For this review, take the finished solid that the model builds, in its own axes (mm). A direction names the side the tool comes from. Round coordinates to 2 decimals unless told otherwise and drop trailing zeros. Order: outer loops, then holes, each group sorted by start corner. A loop starts at its lowest first (then second) coordinate and runs counter-clockwise, first axis right, second up. Notation, with made-up numbers: M -25.75,78.25 L 16.25,78.25 A34 ccw 16.25,111.25 Z; hole C -26,-5 d9. An arc over 180 degrees is marked long. Write item = value, one per line. Start each with the question number.
from build123d import *

# Parameters (mm, degrees)
F0_R     = 1.75
F1_DEPTH = 2


with BuildPart() as f1:
    # F0 (on Front) → F1 (new body)
    with BuildSketch(Plane.XZ):
        with BuildLine():
            Line((13.0079, -4.880859), (15.948683, -2.84605))
            ThreePointArc((15.948683, -2.84605), (17.84605, 0.948683), (14.051317, 2.84605))
            Line((14.051317, 2.84605), (1.581139, -1.310676))
            ThreePointArc((1.581139, -1.310676), (0, -1.56726), (-1.581139, -1.310676))
            Line((-1.581139, -1.310676), (-14.051317, 2.84605))
            ThreePointArc((-14.051317, 2.84605), (-17.84605, 0.948683), (-15.948683, -2.84605))
            Line((-15.948683, -2.84605), (-13.0079, -4.880859))
            ThreePointArc((-13.0079, -4.880859), (-9.695273, -8.626463), (-8.5, -13.481807))
            Line((-8.5, -13.481807), (-8.5, -24))
            ThreePointArc((-8.5, -24), (-8.207107, -24.707107), (-7.5, -25))
            Line((-7.5, -25), (0, -25))
            Line((0, -25), (7.5, -25))
            ThreePointArc((7.5, -25), (8.207107, -24.707107), (8.5, -24))
            Line((8.5, -24), (8.5, -13.481807))
            ThreePointArc((8.5, -13.481807), (9.695273, -8.626463), (13.0079, -4.880859))
        make_face()
        with Locations((-15, 0)):
            Circle(F0_R, mode=Mode.SUBTRACT)
        with Locations((0, -5)):
            Circle(F0_R, mode=Mode.SUBTRACT)
        with Locations((15, 0)):
            Circle(F0_R, mode=Mode.SUBTRACT)
    extrude(amount=F1_DEPTH)


solid = f1.part
(1) We need section C-C, the plane z = 0. Write out the cut boundary in (x, y).
(2) We need section A-A, the plane y = -1.65. Write out the cut boundary in (x, z).
(3) We need section B-B, the plane x = -15. Write out the cut boundary in (y, z), then the cut area to 3 significant figures.
(4) For line 1 along X through (y, z) = (-0.95, -16); line 2 along Z through (x, y) = (-15, -0.35); line 3 along X through (y, z) = (-1.5, -4.5), list the stretches that pass through material, from the lowest coordinate up.
(5) For faces 5 (the cylindrical face through (8.199, -0.986, -24.715)), 6 (the flat face through (-8.5, -1, -19)), 7 (the flat face through (7.904, -0.986, 0.797)), list the 3-axis set-ups (+Z, -Z, +X, -X, +Y, -Y) from which the entire face can be reached by the end or side of a thin tool; tool diameter is ignored.
(6) Insertion check: pin 1 (1 mm diameter, centred on y = -1.5, z = -17, fed in from -X). The pin has a flat end and moves straight along its axis. Give the tip position at first contact, or say it passes through.
(7) Draft analysis for pull direction X (two halves, no side actions). For faces 1 (the cylindrical face through (16.669, -0.986, 0.526)), 2 (the flat face through (8.5, -1, -19)), 3 (the cylindrical face through (-0.38, -0.99, -6.71)), 4 (the cylindrical face through (-9.73, -0.99, -8.56)), state which applies: released by +X, released by -X, zero draft, split by the parting line, or undercut.
(8) We need section D-D, the plane x = 11. Write out the cut boundary in (y, z), then the cut area to 3 significant figures.
Values:
q1.outline = M -18,-2 L -16.75,-2 L -16.75,0 L -18,0 Z; M -13.25,-2 L -5.51,-2 L -5.51,0 L -13.25,0 Z; M 5.51,-2 L 13.25,-2 L 13.25,0 L 5.51,0 Z; M 16.75,-2 L 18,-2 L 18,0 L 16.75,0 Z
q2.outline = M -15.95,-2.85 L -13.01,-4.88 A10.46 cw -8.5,-13.48 L -8.5,-24 A1 ccw -7.5,-25 L 7.5,-25 A1 ccw 8.5,-24 L 8.5,-13.48 A10.46 cw 13.01,-4.88 L 15.95,-2.85 A3 ccw 14.05,2.85 L 1.58,-1.31 A5 cw -1.58,-1.31 L -14.05,2.85 A3 ccw Z; hole C -15,0 d3.5; hole C 0,-5 d3.5; hole C 15,0 d3.5
q3.outline = M -2,-3.5 L 0,-3.5 L 0,-1.75 L -2,-1.75 Z; M -2,1.75 L 0,1.75 L 0,3 L -2,3 Z
q3.area = 6.00 mm²
q4.line_1 = -8.5 to 8.5
q4.line_2 = -3.5 to -1.75, 1.75 to 3
q4.line_3 = -13.56 to -1.68, 1.68 to 13.56
q5.face_5 = -Z, +X, +Y, -Y
q5.face_6 = -Z, -X, +Y, -Y
q5.face_7 = +Z, +Y, -Y
q6.pin_1 = -8.5
q7.face_1 = undercut
q7.face_2 = released by +X
q7.face_3 = undercut
q7.face_4 = released by -X
q8.outline = M -2,-6.7 L 0,-6.7 L 0,1.83 L -2,1.83 Z
q8.area = 17.1 mm²
